Design review of the part built by this model. Coordinates are the model's own, in mm. A direction names the side the tool comes from. Give positions to 0.01 mm unless a question says otherwise; leave off trailing zeros. Write each loop counter-clockwise with the first axis right and the second up, starting at its lowest first coordinate (ties: lowest second). Pieces come first, ordered by that corner, then holes. Notation, with made-up numbers: (-25.5, -27.75) -> (10.5, -27.75) arc R19 cw to (10.5, 0.25) -> close; hole circle Ø3 at (6, -18.5). An arc over 180 degrees is marked (long way). Use CSV: the item, a comma, the result in double quotes.
Autodesk Inventor part; units mm, degrees
ref_plane "YZ Plane" through (0, 0, 0) normal (1, 0, 0) x (0, 1, 0)
ref_plane "XZ Plane" through (0, 0, 0) normal (0, 1, 0) x (-1, 0, 0)
ref_plane "XY Plane" through (0, 0, 0) normal (0, 0, 1) x (1, 0, 0)
sketch "Boceto1" plane through (0, 0, 0) normal (0, 1, 0) x (-1, 0, 0)
  line L0 (14, -5) -> (-14, -5)
  line L1 (-14, -5) -> (-14, 5)
  line L2 (-14, 5) -> (14, 5)
  line L3 (14, 5) -> (14, -5)
  point P0 (0, 0)
  point P1 (0, -5)
  point P2 (-14, 0)
  dimension "d0" = 28
  dimension "d1" = 10
extrude "Extrusión1" add sketch "Boceto1" along normal blind 40
sketch "Boceto2" plane through (0, 0, 0) normal (0, -1, 0) x (1, 0, 0)
  point P0 (0, 0)
  point P1 (6, 0)
  point P2 (-6, 0)
  dimension "d19" = 12
  dimension "d20" = 6
hole "Agujero1" at (6, 0, 0) at (-6, 0, 0) direction (0, 1, 0) diameter 3.242 depth 11.8 tip angle 118
sketch "Boceto3" plane through (-14, 0, 5) normal (0, 0, 1) x (1, 0, 0)
  line L0 (0, 0) -> (28, 0)
  point P0 (14, 0)
  point P1 (14, 28)
  point P2 (14, 0)
  dimension "d11" = 28
hole "Agujero2" at (0, 28, 5) direction (0, 0, -1) diameter 6.647 end through all
sketch "Boceto4" plane through (-14, 0, 5) normal (0, 0, 1) x (1, 0, 0)
  circle A0 centre (14, 10) radius 2.5
  line L0 (0, 0) -> (28, 0)
  point P0 (14, 0)
  point P1 (14, 0)
  dimension "d21" = 5
  dimension "d22" = 10
extrude "Extrusión2" cut sketch "Boceto4" against normal blind 10
properties part number "Guia sujecion centellador"
(1) Take a section at C-C (z = 3.5). Write out the cut boundary in (x, y), then the cut area to 3 significant figures.
Established:
outline,"(-14, 0) -> (14, 0) -> (14, 40) -> (-14, 40) -> close; hole circle Ø6.65 at (0, 28); hole circle Ø5 at (0, 10)"
area,"1,070 mm2"
(2) Take a section at A-A (y = 10). Write out the cut boundary in (x, z), then the cut area to 3 significant figures.
Established:
outline,"(-14, -5) -> (-2.5, -5) -> (-2.5, 5) -> (-14, 5) -> close; (2.5, -5) -> (14, -5) -> (14, 5) -> (2.5, 5) -> close; hole circle Ø3.24 at (-6, 0); hole circle Ø3.24 at (6, 0)"
area,"213 mm2"
(3) For line 1 along X through (y, z) = (3.25, 0); line 2 along Y through (x, z) = (-2, -4.25); line 3 along X through (y, z) = (28, -0.5), list the stretches that pass through material, from the lowest coordinate up. Write a range as [from, to].
Established:
line 1,"x = [-14, -7.62], [-4.38, 4.38], [7.62, 14]"
line 2,"y = [0, 8.5], [11.5, 25.35], [30.65, 40]"
line 3,"x = [-14, -3.32], [3.32, 14]"
(4) Tool access review of faces 1 (the face through (0, 0, 0)), 2 (the face through (7.438, 5.983, -0.748)): name each direction out of +Z, -Z, +X, -X, +Y, -Y from which nothing blocks a thin tool from reaching the whole face with its end or side.
Established:
face 1,"+Z, -Z, +X, -X, -Y"
face 2,"-Y"
(5) Clearance check with a flat-ended pin moving along its axis: pin 1 (5.5 mm diameter, centred on x = 0, y = 28, fed in from +Z). State where the tip first meets the part, or that it passes through.
Established:
pin 1,"passes through"
(6) Mouldability with a two-part tool opening along Z and no side actions: class faces 3 (the face through (2.02, 30.64, -0.07)), 4 (the face through (6.279, 12.605, 0.037)), 5 (the face through (0, 20, -5)), 6 (the face through (-4.418, 5.983, 0.351)) as +Z half, -Z half, draft (parallel to the pull), parting line (faces both ways), or undercut.
Established:
face 3,"draft"
face 4,"undercut"
face 5,"-Z half"
face 6,"undercut"
(7) Take a section at D-D (y = 30.5). Write out the cut boundary in (x, z).
Established:
outline,"(-14, -5) -> (-2.19, -5) -> (-2.19, 5) -> (-14, 5) -> close; (2.19, -5) -> (14, -5) -> (14, 5) -> (2.19, 5) -> close"
(8) Take a section at B-B (x = 0). Write out the cut boundary in (y, z), then the cut area to 3 significant figures.
Established:
outline,"(0, -5) -> (7.5, -5) -> (7.5, 5) -> (0, 5) -> close; (12.5, -5) -> (24.68, -5) -> (24.68, 5) -> (12.5, 5) -> close; (31.32, -5) -> (40, -5) -> (40, 5) -> (31.32, 5) -> close"
area,"284 mm2"
